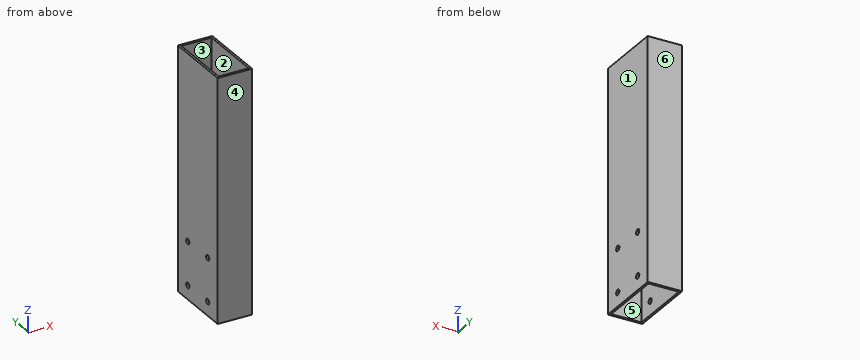
Autodesk Inventor part; units mm, degrees
ref_plane "YZ Plane" through (0, 0, 0) normal (1, 0, 0) x (0, 1, 0)
ref_plane "XZ Plane" through (0, 0, 0) normal (0, 1, 0) x (-1, 0, 0)
ref_plane "XY Plane" through (0, 0, 0) normal (0, 0, 1) x (1, 0, 0)
sketch "Sketch1" plane through (0, 0, 0) normal (0, 0, 1) x (1, 0, 0)
  line L0 (0, 0) -> (25.4, 0)
  line L1 (25.4, 0) -> (25.4, 50.8)
  line L2 (25.4, 50.8) -> (0, 50.8)
  line L3 (0, 50.8) -> (0, 0)
  line L4 (23.8125, 49.2125) -> (23.8125, 1.5875)
  line L5 (23.8125, 1.5875) -> (1.5875, 1.5875)
  line L6 (1.5875, 1.5875) -> (1.5875, 49.2125)
  line L7 (1.5875, 49.2125) -> (23.8125, 49.2125)
  dimension "d0" = 25.4
  dimension "d1" = 50.8
  dimension "d2" = 1.5875
extrude "Extrusion1" add sketch "Sketch1" along normal blind 177.8
sketch "Sketch2" plane through (25.4, 0, 0) normal (1, 0, 0) x (0, 0, -1)
  line L0 (0, 1.5875) -> (0, 49.2125) construction
  line L1 (0, 25.4) -> (0, 38.1) construction
  line L2 (0, 38.1) -> (-10.2108, 38.1) construction
  line L3 (-10.2108, 38.1) -> (-10.2108, 12.7) construction
  line L4 (-10.2108, 12.7) -> (-41.9608, 12.7) construction
  line L5 (-41.9608, 12.7) -> (-41.9608, 38.1) construction
  circle A0 centre (-10.2108, 38.1) radius 2.0193
  circle A1 centre (-10.2108, 12.7) radius 2.0193
  circle A2 centre (-41.9608, 12.7) radius 2.0193
  circle A3 centre (-41.9608, 38.1) radius 2.0193
  point P0 (0, 0)
  dimension "d5" = 12.7
  dimension "d6" = 10.2108
  dimension "d7" = 25.4
  dimension "d9" = 31.75
  dimension "d10" = 4.0386
extrude "Extrusion2" cut sketch "Sketch2" against normal blind 177.8
properties part number "1x2 Placeholder"
Part model, mm, in its own coordinate system. Face numbers are marked on the shaded views. A direction names the side the tool comes from. Round coordinates to 2 decimals unless told otherwise and drop trailing zeros. Write each loop counter-clockwise with the first axis right and the second up, starting at its lowest first coordinate (ties: lowest second). Pieces come first, ordered by that corner, then holes. Notation, with made-up numbers: (84.25, 13) -> (101.25, 13) arc R8 cw to (101.25, 20) -> close; hole circle Ø8 at (32.5, 48.25). An arc over 180 degrees is marked (long way). Return JSON: item names as keys, results as strings. Group by question number.
Q1. Which spindle directions (+Z, -Z, +X, -X, +Y, -Y) get a long thin tool onto all of the face, cutting with end or side? Do the marked faces 1 and 2. Say none if no direction does.
Q2. Probe L1, parallel to X at y = 20, z = 21.5; L2, parallel to Y at x = 6.25, z = 153. List the from-to ranges inside material, lowest first. Write a range as [from, to].
Q3. Saw through at C-C on x = 17.5. Write the cut outline in (y, z), plus the area to 3 significant figures.
Q4. Saw through at A-A on z = 88. Write the cut outline in (x, y).
Q5. Saw through at B-B on y = 7. Write the cut outline in (x, z), plus the area to 3 significant figures.
Q6. Mould opens along Y. For the marked faces 3, 4, 5 and 6 say: pulls with the +Y half, pulls with the -Y half, needs draft (parallel to the pull), parting line crosses it, or undercut.
Answer:
{
 "1": {"face 1": "+Z, -Z, +X, +Y, -Y", "face 2": "+Z, -Z"},
 "2": {"L1": "[0, 1.59], [23.81, 25.4]", "L2": "[0, 1.59], [49.21, 50.8]"},
 "3": {"outline": "(0, 0) -> (1.59, 0) -> (1.59, 177.8) -> (0, 177.8) -> close; (49.21, 0) -> (50.8, 0) -> (50.8, 177.8) -> (49.21, 177.8) -> close", "area": "565 mm2"},
 "4": {"outline": "(0, 0) -> (25.4, 0) -> (25.4, 50.8) -> (0, 50.8) -> close; hole (1.59, 1.59) -> (23.81, 1.59) -> (23.81, 49.21) -> (1.59, 49.21) -> close"},
 "5": {"outline": "(0, 0) -> (1.59, 0) -> (1.59, 177.8) -> (0, 177.8) -> close; (23.81, 0) -> (25.4, 0) -> (25.4, 177.8) -> (23.81, 177.8) -> close", "area": "565 mm2"},
 "6": {"face 3": "undercut", "face 4": "pulls with the -Y half", "face 5": "undercut", "face 6": "pulls with the +Y half"}
}
